from build123d import *

# Parameters (mm, degrees)
SKETCH_1_W          = 136
SKETCH_1_H          = 55
EXTRUDE_1_DEPTH     = 2
SKETCH_2_R          = 1.525
CUT_EXTRUDE_1_DEPTH = 10
SKETCH_3_W          = 20
SKETCH_3_H          = 20
CUT_EXTRUDE_2_DEPTH = 22
FILLET_1_R          = 2
CUT_EXTRUDE_3_DEPTH = 22
EXTRUDE_2_DEPTH     = 2
SKETCH_6_W          = 8
SKETCH_6_H          = 14.5
CUT_EXTRUDE_4_DEPTH = 2
EXTRUDE_3_DEPTH     = 2
FILLET_2_R          = 2
FILLET_3_R          = 2
SKETCH_8_R          = 1.525
CUT_EXTRUDE_5_DEPTH = 10


with BuildPart() as part:
    # 草图1 → 凸台-拉伸1 (new body)
    with BuildSketch(Plane.XY):
        Rectangle(SKETCH_1_W, SKETCH_1_H)
    extrude(amount=EXTRUDE_1_DEPTH)

    # 草图2 → 切除-拉伸1 (cut)
    with BuildSketch(Plane(origin=(0, 0, 0), x_dir=(-1, 0, 0), z_dir=(0, 0, -1))):
        with Locations((59.9, -17.8)):
            Circle(SKETCH_2_R)
        with Locations((65, 19.5)):
            Circle(SKETCH_2_R)
    cut_extrude_1 = extrude(amount=-CUT_EXTRUDE_1_DEPTH, mode=Mode.SUBTRACT)

    # 镜向1: 切除-拉伸1 across plane
    add(cut_extrude_1.mirror(Plane(origin=(0, 0, 0), x_dir=(0, 0, 1), z_dir=(1, 0, 0))), mode=Mode.SUBTRACT)

    # 草图3 → 切除-拉伸2 (cut)
    with BuildSketch(Plane(origin=(0, 0, 0), x_dir=(-1, 0, 0), z_dir=(0, 0, -1))):
        with Locations((0, -27.5)):
            Rectangle(SKETCH_3_W, SKETCH_3_H)
    extrude(amount=-CUT_EXTRUDE_2_DEPTH, mode=Mode.SUBTRACT)

    # 圆角1
    fillet_1_edges = [part.edges().sort_by_distance(p)[0] for p in [
        (10, -27.5, 1),
        (10, -17.5, 1),
        (-10, -27.5, 1),
        (-10, -17.5, 1),
    ]]
    fillet(fillet_1_edges, radius=FILLET_1_R)

    # 草图4 → 切除-拉伸3 (cut)
    with BuildSketch(Plane.XY.offset(2)):
        Polygon((-61.236241819, 21.5), (-55.356885251, -21.5), (-15, -21.5), (-15, 21.5), align=None)
    cut_extrude_3 = extrude(amount=-CUT_EXTRUDE_3_DEPTH, mode=Mode.SUBTRACT)

    # 草图5 → 凸台-拉伸2 (add)
    with BuildSketch(Plane.XY.offset(2)):
        Polygon((-61.236241819, 21.5), (-38.11812091, -21.5), (-33.576673053, -21.5), (-56.694793962, 21.5), align=None)
        Polygon((-38.11812091, 21.5), (-15, -21.5), (-19.541447857, -21.5), (-42.659568766, 21.5), align=None)
    extrude_2 = extrude(amount=-EXTRUDE_2_DEPTH)

    # 镜向3: 切除-拉伸3, 凸台-拉伸2 across plane
    add(cut_extrude_3.mirror(Plane(origin=(0, 0, 0), x_dir=(0, 0, 1), z_dir=(1, 0, 0))), mode=Mode.SUBTRACT)
    add(extrude_2.mirror(Plane(origin=(0, 0, 0), x_dir=(0, 0, 1), z_dir=(1, 0, 0))))

    # 草图6 → 切除-拉伸4 (cut)
    with BuildSketch(Plane.XY.offset(2)):
        with Locations((-6, 14.25)):
            Rectangle(SKETCH_6_W, SKETCH_6_H)
        with Locations((6, 14.25)):
            Rectangle(SKETCH_6_W, SKETCH_6_H)
        with Locations((6, -4.25)):
            Rectangle(SKETCH_6_W, SKETCH_6_H)
        with Locations((-6, -4.25)):
            Rectangle(SKETCH_6_W, SKETCH_6_H)
    extrude(amount=-CUT_EXTRUDE_4_DEPTH, mode=Mode.SUBTRACT)

    # 草图7 → 凸台-拉伸3 (add)
    with BuildSketch(Plane(origin=(0, 0, 0), x_dir=(-1, 0, 0), z_dir=(0, 0, -1))):
        with BuildLine():
            Line((-16.458323102, 22.868683211), (-56.815208352, -20.131316789))
            ThreePointArc((-56.815208352, -20.131316789), (-56.725568462, -22.958323102), (-53.898562149, -22.868683211))
            Line((-53.898562149, -22.868683211), (-13.541676898, 20.131316789))
            ThreePointArc((-13.541676898, 20.131316789), (-13.631316789, 22.958323102), (-16.458323102, 22.868683211))
        make_face()
    extrude_3 = extrude(amount=-EXTRUDE_3_DEPTH)

    # 镜向4: 凸台-拉伸3 across plane
    add(extrude_3.mirror(Plane(origin=(0, 0, 0), x_dir=(0, 0, 1), z_dir=(1, 0, 0))))

    # 圆角2
    fillet_2_edges = [part.edges().sort_by_distance(p)[0] for p in [
        (-38.11812091, -21.5, 1),
        (-33.576673053, -21.5, 1),
        (-56.694793962, 21.5, 1),
        (-19.541447857, -21.5, 1),
        (-38.11812091, 21.5, 1),
        (-42.659568766, 21.5, 1),
        (61.236241819, 21.5, 1),
        (15, -21.5, 1),
        (56.694793962, 21.5, 1),
        (38.11812091, -21.5, 1),
        (33.576673053, -21.5, 1),
        (38.11812091, 21.5, 1),
        (42.659568766, 21.5, 1),
        (19.541447857, -21.5, 1),
        (-2, 3, 1),
        (-2, -11.5, 1),
        (-10, -11.5, 1),
        (-10, 3, 1),
        (2, -11.5, 1),
        (10, -11.5, 1),
        (10, 3, 1),
        (2, 3, 1),
        (2, 7, 1),
        (10, 7, 1),
        (10, 21.5, 1),
        (2, 21.5, 1),
        (-2, 7, 1),
        (-2, 21.5, 1),
        (-10, 21.5, 1),
        (-10, 7, 1),
        (30.69728876, 7.697157473, 1),
        (28.699332342, 3.980933031, 1),
        (52.614008864, -21.5, 1),
        (43.397642893, -11.680021717, 1),
        (40.510227812, -8.603499639, 1),
        (15, 18.577482964, 1),
        (55.705666805, -18.949107453, 1),
        (45.39559931, -7.963797276, 1),
        (42.50818423, -4.887275198, 1),
        (17.742876387, 21.5, 1),
        (31.586747423, 0.904410953, 1),
        (33.58470384, 4.620635395, 1),
        (-30.69728876, 7.697157473, 1),
        (-28.699332342, 3.980933031, 1),
        (-52.614008864, -21.5, 1),
        (-15, 18.577482964, 1),
        (-43.397642893, -11.680021717, 1),
        (-40.510227812, -8.603499639, 1),
        (-31.586747423, 0.904410953, 1),
        (-17.742876387, 21.5, 1),
        (-55.705666805, -18.949107453, 1),
        (-45.39559931, -7.963797276, 1),
        (-42.50818423, -4.887275198, 1),
        (-33.58470384, 4.620635395, 1),
        (-61.236241819, 21.5, 1),
        (-15, -21.5, 1),
    ]]
    fillet(fillet_2_edges, radius=FILLET_2_R)

    # 圆角3
    fillet_3_edges = [part.edges().sort_by_distance(p)[0] for p in [
        (68, -27.5, 1),
        (-68, -27.5, 1),
        (-68, 27.5, 1),
        (68, 27.5, 1),
    ]]
    fillet(fillet_3_edges, radius=FILLET_3_R)

    # 草图8 → 切除-拉伸5 (cut)
    with BuildSketch(Plane(origin=(0, 0, 0), x_dir=(-1, 0, 0), z_dir=(0, 0, -1))):
        with Locations((53, 24.5)):
            Circle(SKETCH_8_R)
        with Locations((35, 24.5)):
            Circle(SKETCH_8_R)
    cut_extrude_5 = extrude(amount=-CUT_EXTRUDE_5_DEPTH, mode=Mode.SUBTRACT)

    # 镜向5: 切除-拉伸5 across plane
    add(cut_extrude_5.mirror(Plane(origin=(0, 0, 0), x_dir=(0, 0, 1), z_dir=(1, 0, 0))), mode=Mode.SUBTRACT)


solid = part.part
Here's how the part is built. I have some questions about the finished solid (model axes, mm). Coordinates: 2 decimals unless noted, no trailing zeros.
Item 1: If I drill on line 1 (Y direction, x = 65, z = 1.25) (3 decimals); line 2 (X direction, y = -24, z = 0.75); line 3 (X direction, y = -21, z = 0.2), over which ranges is the centre line in solid material (lowest first)?
Item 2: I want a section at A-A on z = 1. Count the separate pieces of the cut face and the enclosed holes in it, and give its area (3 significant figures).
Item 3: If we mould it in two halves opening along Y, with no side actions, what happens to faces 1 (the flat face through (1, 0, 0)), 2 (the cylindrical face through (66.4, 18.9, 1))? For each: +Y half, -Y half, draft (parallel to the pull), parting line (faces both ways), or undercut.
Findings below:
1. line 1: y = -27.5 to 17.975, 21.025 to 27.5
1. line 2: x = -68 to -10, 10 to 68
1. line 3: x = -68 to -49.32, -40.14 to -33.7, -21.56 to -10, 10 to 21.56, 33.7 to 40.14, 49.32 to 68
2. separate pieces: 1
2. enclosed holes: 24
2. area: 4,340 mm2
3. face 1: draft
3. face 2: undercut
